The listing builds one solid part. Answer for the finished solid, in the listing's coordinates (mm). Give positions to 0.01 mm unless a question says otherwise; leave off trailing zeros. Order: outer loops, then holes, each group sorted by start corner. A loop starts at its lowest first (then second) coordinate and runs counter-clockwise, first axis right, second up. Notation, with made-up numbers: M 11,-25 L 43,-25 A32 cw 43,8 Z; hole C -25,52.25 d11. An arc over 180 degrees is marked long. Answer as a JSON object with one key per item and string values. Group by question number.
```python
from build123d import *

# Parameters (mm, degrees)
ESQUISSE1_W                  = 600
ESQUISSE1_H                  = 580
BOSS_EXTRU_1_DEPTH           = 38
ENL_V_MAT_EXTRU_1_DEPTH      = 836.370576451
ENL_V_MAT_EXTRU_1_DEPTH_BACK = 836.370576451
ESQUISSE2_R                  = 50
ESQUISSE3_R                  = 62
ENL_V_MAT_EXTRU_3_DEPTH      = 10
ESQUISSE4_W                  = 600
ESQUISSE4_H                  = 30
ENL_V_MAT_EXTRU_4_DEPTH      = 12.8
ESQUISSE5_W                  = 30
ESQUISSE5_H                  = 280
ENL_V_MAT_EXTRU_5_DEPTH      = 12.8


with BuildPart() as part:
    # Esquisse1 → Boss.-Extru.1 (new body)
    with BuildSketch(Plane.XY):
        with Locations((300, 290)):
            Rectangle(ESQUISSE1_W, ESQUISSE1_H)
    extrude(amount=BOSS_EXTRU_1_DEPTH)

    # Esquisse2 → Enlèv. mat.-Extru.1 (cut, two sides: drawn at the far end of the back side and taken through both)
    with BuildSketch(Plane.XY.offset(38).offset(-ENL_V_MAT_EXTRU_1_DEPTH_BACK)):
        with Locations((300, 290)):
            Circle(ESQUISSE2_R)
    extrude(amount=ENL_V_MAT_EXTRU_1_DEPTH + ENL_V_MAT_EXTRU_1_DEPTH_BACK, mode=Mode.SUBTRACT)

    # Esquisse3 → Enlèv. mat.-Extru.3 (cut)
    with BuildSketch(Plane.XY):
        with Locations((300, 290)):
            Circle(ESQUISSE3_R)
    extrude(amount=ENL_V_MAT_EXTRU_3_DEPTH, mode=Mode.SUBTRACT)

    # Esquisse4 → Enlèv. mat.-Extru.4 (cut)
    with BuildSketch(Plane(origin=(0, 0, 0), x_dir=(-1, 0, 0), z_dir=(0, 0, -1))):
        with Locations((-300, 405)):
            Rectangle(ESQUISSE4_W, ESQUISSE4_H)
        with Locations((-300, 525)):
            Rectangle(ESQUISSE4_W, ESQUISSE4_H)
    extrude(amount=-ENL_V_MAT_EXTRU_4_DEPTH, mode=Mode.SUBTRACT)

    # Esquisse5 → Enlèv. mat.-Extru.5 (cut)
    with BuildSketch(Plane(origin=(0, 0, 0), x_dir=(-1, 0, 0), z_dir=(0, 0, -1))):
        with Locations((-65, 140)):
            Rectangle(ESQUISSE5_W, ESQUISSE5_H)
        with Locations((-535, 140)):
            Rectangle(ESQUISSE5_W, ESQUISSE5_H)
    extrude(amount=-ENL_V_MAT_EXTRU_5_DEPTH, mode=Mode.SUBTRACT)


solid = part.part
```
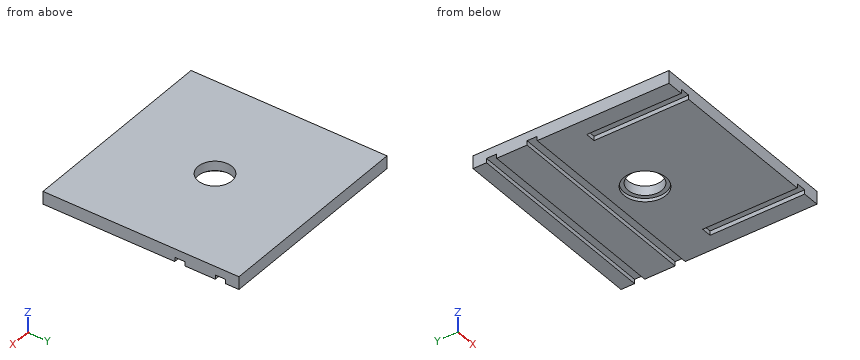
Item 1: Section C-C (z = 26) is taken. Determine the outline of the cut face in (x, y), and give its area (3 significant figures).
Item 2: Consider probe 1 along X at (y, z) = (215.5, 5); probe 2 along Y at (x, z) = (395.5, 2); probe 3 along Y at (x, z) = (300, 2). Determine where each line is inside the solid, lowest interval first. Write a range as from..to.
Item 3: Flat-ended cylindrical pins translate along their axes: P1, Ø4, axis at x = 415, z = 7, coming from the -Y side; P2, Ø9, axis at x = 189, y = 526.5, coming from the -Z side; P3, Ø6.5, axis at x = 531.5, z = 6, coming from the -Y side. Find the tip coordinate at first contact, or state that the pin passes through.
Item 4: Section A-A (x = 300) is taken. Determine the outline of the cut face in (y, z).
Item 5: Section B-B (y = 290) is taken. Determine the outline of the cut face in (x, z), and give its area (3 significant figures).
Item 6: Section D-D (y = 70.5) is taken. Determine the outline of the cut face in (x, z).
Values found:
{
 "1": {"outline": "M 0,0 L 600,0 L 600,580 L 0,580 Z; hole C 300,290 d100", "area": "340,000 mm^2"},
 "2": {"probe 1": "x = 0..50, 80..520, 550..600", "probe 2": "y = 0..390, 420..510, 540..580", "probe 3": "y = 0..228, 352..390, 420..510, 540..580"},
 "3": {"P1": "stops at y = 0", "P2": "stops at z = 12.8", "P3": "stops at y = 280"},
 "4": {"outline": "M 0,0 L 228,0 L 228,10 L 240,10 L 240,38 L 0,38 Z; M 340,10 L 352,10 L 352,0 L 390,0 L 390,12.8 L 420,12.8 L 420,0 L 510,0 L 510,12.8 L 540,12.8 L 540,0 L 580,0 L 580,38 L 340,38 Z"},
 "5": {"outline": "M 0,0 L 238,0 L 238,10 L 250,10 L 250,38 L 0,38 Z; M 350,10 L 362,10 L 362,0 L 600,0 L 600,38 L 350,38 Z", "area": "18,800 mm^2"},
 "6": {"outline": "M 0,0 L 50,0 L 50,12.8 L 80,12.8 L 80,0 L 520,0 L 520,12.8 L 550,12.8 L 550,0 L 600,0 L 600,38 L 0,38 Z"}
}
